The drawing under review shows one solid part. Ordinate dimensions are in mm from its lowest x, y, z. Round coordinates to 2 decimals unless told otherwise and drop trailing zeros. Order: outer loops, then holes, each group sorted by start corner. A loop starts at its lowest first (then second) coordinate and runs counter-clockwise, first axis right, second up. Notation, with made-up numbers: M -34.5,21 L -19.5,21 A10 cw -19.5,27 Z; hole C -17,0.25 d8. An arc over 180 degrees is marked long. Use a Markdown table: item, result.
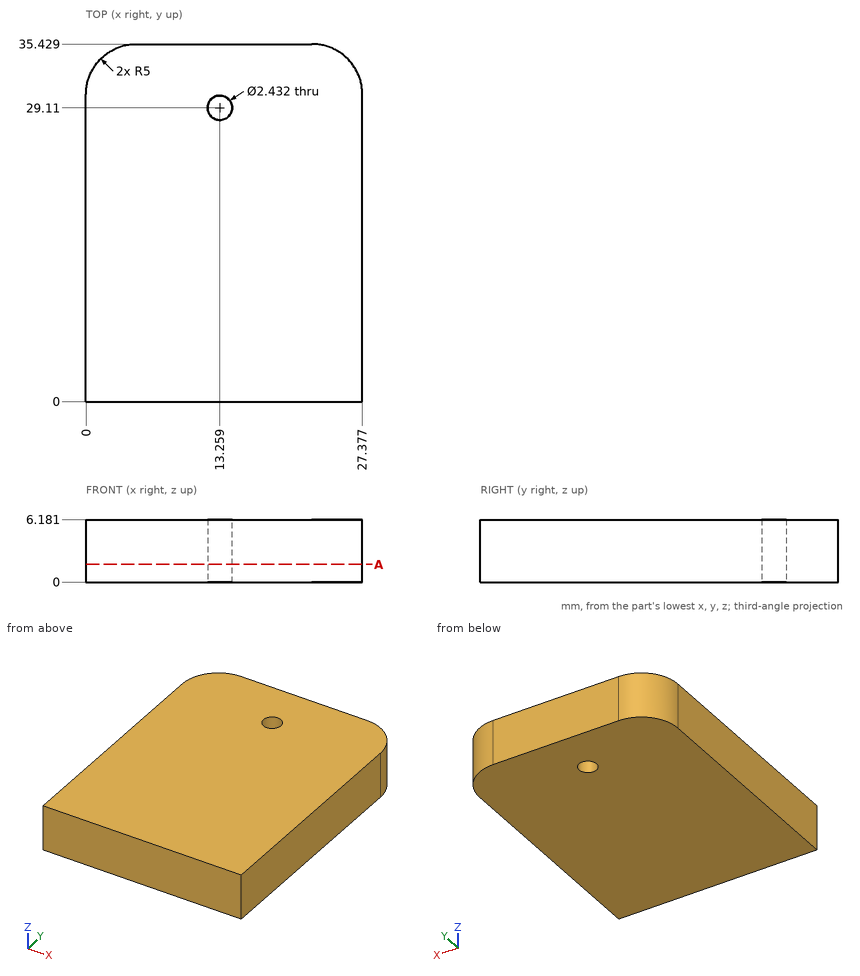
Q1. Clearance check with a flat-ended pin moving along its axis: pin 1 (10 mm diameter, centred on x = 20, y = 17, fed in from -Z). State where the tip first meets the part, or that it passes through.
Determined:
| item | result |
|---|---|
| pin 1 | stops at z = 0 |
Q2. Wall thickness on line 1 along X through (y, z) = (29, 2); line 2 along Y through (x, z) = (13.5, 4.5); line 3 along X through (y, z) = (28.5, 3.75) (1 decimal): over which ranges is each line inside the solid? List them lowest first. Write a range as [from, to].
Determined:
| item | result |
|---|---|
| line 1 | x = [0, 12.05], [14.47, 27.38] |
| line 2 | y = [0, 27.92], [30.3, 35.43] |
| line 3 | x = [0, 12.2], [14.3, 27.4] |
Q3. Add section A-A (z = 1.75). Write out the cut boundary in (x, y) (1 decimal).
Determined:
| item | result |
|---|---|
| outline | M 0,0 L 27.4,0 L 27.4,30.4 A5 ccw 22.4,35.4 L 5,35.4 A5 ccw 0,30.4 Z; hole C 13.3,29.1 d2.4 |
